from build123d import *

# Parameters (mm, degrees)
BOSS_EXTRUDE1_DEPTH      = 9.5
BOSS_EXTRUDE1_DEPTH_BACK = 9.5
SKETCH1_R                = 21
SKETCH5_R                = 14.7
CUT_EXTRUDE3_DEPTH       = 1
SKETCH6_R                = 10.65
CUT_EXTRUDE4_DEPTH       = 11.6
SKETCH7_R                = 3.925
BOSS_EXTRUDE2_DEPTH      = 6.08
CUT_EXTRUDE1_DEPTH       = 36.256205128
CUT_EXTRUDE2_START       = -4.5
SKETCH4_R                = 14.7
CUT_EXTRUDE2_DEPTH       = 4.5


with BuildPart() as part:
    # Sketch1 → Boss-Extrude1 (new, two sides: drawn at the far end of the back side and taken through both)
    with BuildSketch(Plane(origin=(0, 0, 0), x_dir=(0, 0, -1), z_dir=(1, 0, 0)).offset(-BOSS_EXTRUDE1_DEPTH_BACK)):
        Circle(SKETCH1_R)
    extrude(amount=BOSS_EXTRUDE1_DEPTH + BOSS_EXTRUDE1_DEPTH_BACK)

    # Sketch5 → Cut-Extrude3 (cut)
    with BuildSketch(Plane(origin=(9.5, 0, 0), x_dir=(0, 0, -1), z_dir=(1, 0, 0))):
        Circle(SKETCH5_R)
    extrude(amount=-CUT_EXTRUDE3_DEPTH, mode=Mode.SUBTRACT)

    # Sketch6 → Cut-Extrude4 (cut)
    with BuildSketch(Plane(origin=(8.5, 0, 0), x_dir=(0, 0, -1), z_dir=(1, 0, 0))):
        Circle(SKETCH6_R)
    extrude(amount=-CUT_EXTRUDE4_DEPTH, mode=Mode.SUBTRACT)

    # Sketch7 → Boss-Extrude2 (add)
    with BuildSketch(Plane(origin=(-3.1, 0, 0), x_dir=(0, 0, -1), z_dir=(1, 0, 0))):
        Circle(SKETCH7_R)
    extrude(amount=BOSS_EXTRUDE2_DEPTH)

    # Sketch2 → Cut-Extrude1 (cut, through all)
    with BuildSketch(Plane(origin=(9.5, 0, 0), x_dir=(0, 0, -1), z_dir=(1, 0, 0))):
        with BuildLine():
            Line((-1.118033989, -1), (1.118033989, -1))
            ThreePointArc((1.118033989, -1), (1.472757251, 0.284580535), (0.665, 1.344535236))
            Line((0.665, 1.344535236), (0.665, 8.879705587))
            Line((0.665, 8.879705587), (-0.665, 8.879705587))
            Line((-0.665, 8.879705587), (-0.665, 1.344535236))
            ThreePointArc((-0.665, 1.344535236), (-1.472757251, 0.284580535), (-1.118033989, -1))
        make_face()
    extrude(amount=-CUT_EXTRUDE1_DEPTH, mode=Mode.SUBTRACT)

    # Sketch4 → Cut-Extrude2 (cut)
    with BuildSketch(Plane.ZY.offset(9.5).offset(CUT_EXTRUDE2_START)):
        with Locations(Location((0, 0, 0), (0, 0, 180))):
            Circle(SKETCH4_R)
    extrude(amount=CUT_EXTRUDE2_DEPTH, mode=Mode.SUBTRACT)


solid = part.part
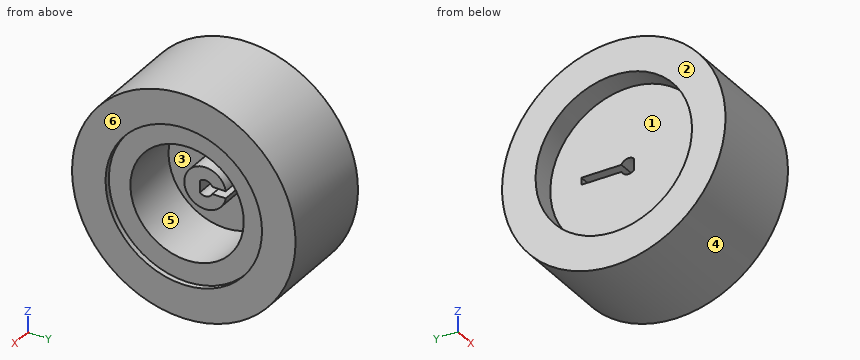
Source: CAD feature listing. Evaluate the final solid. Frame: model axes, mm. Face numbers are marked on the shaded views. A direction names the side the tool comes from. Give positions to 0.01 mm unless a question says otherwise; leave off trailing zeros. Write each loop counter-clockwise with the first axis right and the second up, starting at its lowest first coordinate (ties: lowest second). Pieces come first, ordered by that corner, then holes. Notation, with made-up numbers: M 69.25,-2.75 L 119.25,-2.75 A29 cw 119.25,21.25 Z; hole C -15,6.25 d11. An arc over 180 degrees is marked long. Return JSON: item names as keys, results as strings. Group by question number.
1) Cut plane C-C, the plane z = 0. Output: boundary loops of the cut face in (x, y) (3 decimals).
2) Material intervals for line 1 along Y through (x, z) = (2, 0) (3 decimals); line 2 along Y through (x, z) = (6, 0); line 3 along Z through (x, y) = (0.5, -7), sorted ascending. Write a range as [from, to].
3) Set-up query: the marked faces 1, 2 and 3. Return all of +Z, -Z, +X, -X, +Y, -Y with unobstructed straight access to the full face (end or side cutting, diameter ignored); none if empty.
4) Cut plane D-D, the plane x = -7.5. Output: boundary loops of the cut face in (y, z).
5) Pin query (flat end, axial travel): P1, Ø14.5, axis at y = -7, z = -2, coming from the -X side; P2, Ø6, axis at x = 1, y = -6, coming from the +Z side; P3, Ø2.5, axis at x = 0, y = 4, coming from the -Z side. Return the tip coordinate at first contact, or that it passes through.
6) Cut plane B-B, the plane x = -1.5. Output: boundary loops of the cut face in (y, z) (3 decimals), plus the area to 3 significant figures.
7) Pull-direction query (Y, two-part tool) for the marked faces 4, 5 and 6; classes: pulls with the +Y half, pulls with the -Y half, needs draft (parallel to the pull), parting line crosses it, or undercut.
8) Cut plane A-A, the plane y = 0. Output: boundary loops of the cut face in (x, z) (3 decimals).
Recorded:
{
 "1": {"outline": "M -9.5,-21 L 9.5,-21 L 9.5,-14.7 L 8.5,-14.7 L 8.5,-10.65 L -3.1,-10.65 L -3.1,-3.925 L 2.98,-3.925 L 2.98,-1 L -5,-1 L -5,-14.7 L -9.5,-14.7 Z; M -9.5,14.7 L -5,14.7 L -5,8.88 L -3.1,8.88 L -3.1,10.65 L 8.5,10.65 L 8.5,14.7 L 9.5,14.7 L 9.5,21 L -9.5,21 Z"},
 "2": {"line 1": "y = [-21, -10.65], [-3.925, -1], [10.65, 21]", "line 2": "y = [-21, -10.65], [10.65, 21]", "line 3": "z = [-19.8, -8.03], [8.03, 19.8]"},
 "3": {"face 1": "-X", "face 2": "+Z, -Z, -X, +Y, -Y", "face 3": "+X"},
 "4": {"outline": "C 0,0 d42; hole C 0,0 d29.4"},
 "5": {"P1": "stops at x = -5", "P2": "stops at z = 20.78", "P3": "stops at z = -20.82"},
 "6": {"outline": "C 0,0 d42; M -1,-1.118 L -1,1.118 A1.5 cw 1.345,0.665 L 3.868,0.665 A3.925 ccw long 3.868,-0.665 L 1.345,-0.665 A1.5 cw Z; hole C 0,0 d21.3", "area": "1,070 mm²"},
 "7": {"face 4": "parting line crosses it", "face 5": "undercut", "face 6": "needs draft"},
 "8": {"outline": "M -9.5,-21 L 9.5,-21 L 9.5,-14.7 L 8.5,-14.7 L 8.5,-10.65 L -3.1,-10.65 L -3.1,-3.925 L 2.98,-3.925 L 2.98,-1.5 L -5,-1.5 L -5,-14.7 L -9.5,-14.7 Z; M -9.5,14.7 L -5,14.7 L -5,1.5 L 2.98,1.5 L 2.98,3.925 L -3.1,3.925 L -3.1,10.65 L 8.5,10.65 L 8.5,14.7 L 9.5,14.7 L 9.5,21 L -9.5,21 Z"}
}
